Model file for the job. Use its own axes, mm. A direction names the side the tool comes from. Give positions to 0.01 mm unless a question says otherwise; leave off trailing zeros. Order: outer loops, then holes, each group sorted by start corner. A loop starts at its lowest first (then second) coordinate and runs counter-clockwise, first axis right, second up. Notation, with made-up numbers: (-27.5, -16) -> (-3.5, -16) arc R22 cw to (-3.5, 16) -> close; hole circle Ø8 at (10.5, 29.25). An arc over 180 degrees is marked (long way). Answer in a Markdown table with one row per item. Add a question column.
from build123d import *

# Parameters (mm, degrees)
F0_W     = 80
F0_H     = 50
F1_DEPTH = 27
F2_W     = 76
F2_H     = 46
F3_DEPTH = 25
F4_R     = 3
F5_DEPTH = 2
F6_R     = 1.5
F7_DEPTH = 3
F8_R     = 5
F9_DEPTH = 25
F10_R    = 1.99999


# Not quite as in the source:
# - a fillet or chamfer is up to 0.001 mm smaller than in the source, because OpenCascade refuses the exact size


with BuildPart() as f1:
    # F0 (on Top) → F1 (new body)
    with BuildSketch(Plane.XY):
        Rectangle(F0_W, F0_H)
    extrude(amount=F1_DEPTH)

    # F2 (on face) → F3 (cut)
    with BuildSketch(Plane.XY.offset(27)):
        Rectangle(F2_W, F2_H)
    extrude(amount=-F3_DEPTH, mode=Mode.SUBTRACT)

    # F4 (on face) → F5 (join)
    with BuildSketch(Plane.XY.offset(2)):
        with Locations((-33, 17)):
            Circle(F4_R)
        with Locations((27, 17)):
            Circle(F4_R)
        with Locations((27, -17)):
            Circle(F4_R)
        with Locations((-33, -17)):
            Circle(F4_R)
    extrude(amount=F5_DEPTH)

    # F6 (on face) → F7 (join)
    with BuildSketch(Plane.XY.offset(4)):
        with Locations((-33, 17)):
            Circle(F6_R)
        with Locations((27, 17)):
            Circle(F6_R)
        with Locations((27, -17)):
            Circle(F6_R)
        with Locations((-33, -17)):
            Circle(F6_R)
    extrude(amount=F7_DEPTH)

    # F8 (on face) → F9 (cut)
    with BuildSketch(Plane(origin=(-40, 0, 0), x_dir=(0, -1, 0), z_dir=(-1, 0, 0))):
        with Locations((0, 14)):
            Circle(F8_R)
    extrude(amount=-F9_DEPTH, mode=Mode.SUBTRACT)

    # F10 (radius 2 in the source; OpenCascade refuses exactly that, so slightly less here)
    f10_edges = [f1.edges().sort_by_distance(p)[0] for p in [
        (-38, 23, 14.5),
        (38, 23, 14.5),
        (38, -23, 14.5),
        (-38, -23, 14.5),
        (0, 23, 2),
        (38, 0, 2),
        (0, -23, 2),
        (-38, 0, 2),
    ]]
    fillet(f10_edges, radius=F10_R)


solid = f1.part
Item 1: Saw through at A-A on z = 24. List the corners of the cut face in (x, y).
Item 2: Wall check: line 1 (Y direction, x = 11, z = 18.25); line 2 (X direction, y = 5, z = 22.5); line 3 (Z direction, x = -39.05, y = 0). Give the ranges that are in metal, low to high.
Item 3: Which spindle directions (+Z, -Z, +X, -X, +Y, -Y) get a long thin tool onto all of the face, cutting with end or side? Do faces 1 (the cylindrical face through (-39.01, 1.08, 9.12)), 2 (the cylindrical face through (37.43, 0.29, 2.6)), 3 (the flat face through (-1, 25, 13)). Say none if no direction does.
Item 4: Pin check, flat tips, straight feed: pin 1 Ø3 at (x, y) = (26.5, -15.5) entering from +Z; pin 2 Ø10 at (x, y) = (-25, -1) entering from +Z; pin 3 Ø8 at (y, z) = (0, 14) entering from -X. Stop position of each tip, or through.
Item 5: Saw through at B-B on y = 0. List the corners of the cut face in (x, z).
Item 6: Saw through at D-D on x = -33. List the corners of the cut face in (y, z).
Item 7: Two-plate mould, pull along X, no slides. Class faces 4 (the cylindrical face through (-37.4, 22.43, 15.34)), 5 (the flat face through (40, 0, 13)), 6 (the flat face through (-1, 0, 0)): pulls with the +X half, pulls with the -X half, needs draft (parallel to the pull), parting line crosses it, or undercut.
Evaluation:
| question | item | result |
|---|---|---|
| 1 | outline | (-40, -25) -> (40, -25) -> (40, 25) -> (-40, 25) -> close; hole (-38, -21) arc R2 ccw to (-36, -23) -> (36, -23) arc R2 ccw to (38, -21) -> (38, 21) arc R2 ccw to (36, 23) -> (-36, 23) arc R2 ccw to (-38, 21) -> close |
| 2 | line 1 | y = -25 to -23, 23 to 25 |
| 2 | line 2 | x = -40 to -38, 38 to 40 |
| 2 | line 3 | z = 0 to 9, 19 to 27 |
| 3 | face 1 | -X |
| 3 | face 2 | +Z |
| 3 | face 3 | +Z, -Z, +X, -X, +Y |
| 4 | pin 1 | stops at z = 7 |
| 4 | pin 2 | stops at z = 2 |
| 4 | pin 3 | stops at x = 38 |
| 5 | outline | (-40, 0) -> (40, 0) -> (40, 27) -> (38, 27) -> (38, 4) arc R2 cw to (36, 2) -> (-36, 2) arc R2 cw to (-38, 4) -> (-38, 9) -> (-40, 9) -> close; (-40, 19) -> (-38, 19) -> (-38, 27) -> (-40, 27) -> close |
| 6 | outline | (-25, 0) -> (25, 0) -> (25, 27) -> (23, 27) -> (23, 4) arc R2 cw to (21, 2) -> (20, 2) -> (20, 4) -> (18.5, 4) -> (18.5, 7) -> (15.5, 7) -> (15.5, 4) -> (14, 4) -> (14, 2) -> (-14, 2) -> (-14, 4) -> (-15.5, 4) -> (-15.5, 7) -> (-18.5, 7) -> (-18.5, 4) -> (-20, 4) -> (-20, 2) -> (-21, 2) arc R2 cw to (-23, 4) -> (-23, 27) -> (-25, 27) -> close |
| 7 | face 4 | undercut |
| 7 | face 5 | pulls with the +X half |
| 7 | face 6 | needs draft |
